Can you work these out from the model? Positions are in its coordinate system, mm. Coordinates: 2 decimals unless noted, no trailing zeros. Use one line per item in the form item = value. Start each with the question number.
(1) I'm going to push flat-ended pins straight in: pin 1 (3 mm diameter, centred on x = -27.5, z = 26, fed in from -Y); pin 2 (1.5 mm diameter, centred on x = 9.5, z = 28.5, fed in from +Y); pin 3 (1 mm diameter, centred on x = 28, y = 1, fed in from +Z); pin 4 (3 mm diameter, centred on x = 0.5, z = -1, fed in from +Y). Where does each tip first touch, or does it pass through?
(2) I need wall thicknesses on line 1 (Z direction, x = 0, y = 5.55); line 2 (Z direction, x = -7.5, y = 5.5); line 3 (X direction, y = 5.5, z = -28). Which ranges of each line are inside material? Lowest first, please. Write a range as [from, to].
(3) Thinking about a two-plate mould opening in Z: for faces 1 (the flat face through (0, 3, -6)), 2 (the flat face through (0, 0, 0)), 3 (the cylindrical face through (7.696, 4.219, 34.656)), which applies, released by +Z, released by -Z, zero draft, split by the parting line, or undercut?
Autodesk Inventor part; units mm, degrees
ref_plane "YZ Plane" through (0, 0, 0) normal (1, 0, 0) x (0, 1, 0)
ref_plane "XZ Plane" through (0, 0, 0) normal (0, 1, 0) x (-1, 0, 0)
ref_plane "XY Plane" through (0, 0, 0) normal (0, 0, 1) x (1, 0, 0)
sketch "Sketch1" plane through (0, 0, 0) normal (0, 1, 0) x (-1, 0, 0)
  circle A0 centre (0, 0) radius 32.5
  circle A1 centre (0, 0) radius 35.5
  dimension "d0" = 65
  dimension "d1" = 71
extrude "Extrusion1" add sketch "Sketch1" along normal blind 8
extrude "Extrusion2" add sketch "Sketch1" along normal blind 3 contours A0
fillet "Fillet1" radius 2 2 edges at (35.5, 0, 0) (32.5, 3, 0)
fillet "Fillet2" radius 1.5 2 edges at (32.5, 8, 0) (35.5, 8, 0)
sketch "Sketch2" plane through (0, 3, 0) normal (0, 1, 0) x (1, 0, 0)
  line L0 (-2.5, -2.5) -> (2.5, -2.5)
  line L1 (2.5, -2.5) -> (2.5, 2.5)
  line L2 (2.5, 2.5) -> (-2.5, 2.5)
  line L3 (-2.5, 2.5) -> (-2.5, -2.5)
  line L4 (-2.5, -2.5) -> (2.5, 2.5) construction
  line L5 (2.5, -2.5) -> (-2.5, 2.5) construction
  line L6 (0, -2.5) -> (2.5, 0)
  line L7 (0, -2.5) -> (-2.5, 0)
  circle A0 centre (1.25, 1.25) radius 1.7678
  circle A1 centre (-1.25, 1.25) radius 1.7678
  point P0 (0, 0)
  point P1 (0, 2.5)
  dimension "d8" = 5
  dimension "d9" = 5
extrude "Extrusion3" cut sketch "Sketch2" against normal blind 1 contours L7 A1 A0 L6 | A1 L3 | L3 L2 A0 A1 | A0 A1 L2 L1 | L1 A0 | A1 L2 | A0 A1 | L2 A0
properties part number "Orchid Coaster V3"
Worked out:
q1.pin_1 = through
q1.pin_2 = 3.02
q1.pin_3 = 22.14
q1.pin_4 = 2
q2.line_1 = [-35.5, -32.5], [32.5, 35.5]
q2.line_2 = [-34.7, -31.62], [31.62, 34.7]
q2.line_3 = [-21.82, -16.5], [16.5, 21.82]
q3.face_1 = undercut
q3.face_2 = zero draft
q3.face_3 = split by the parting line
